from build123d import *

# Parameters (mm, degrees)
SKETCH1_W           = 133
SKETCH1_H           = 133
SKETCH1_W_2         = 125
SKETCH1_H_2         = 125
BOSS_EXTRUDE1_DEPTH = 55
SKETCH1_3_W         = 19.05
SKETCH1_3_H         = 19.05
BOSS_EXTRUDE2_DEPTH = 3.175
SKETCH2_W           = 133
SKETCH2_H           = 133
SKETCH2_R           = 2.5
BOSS_EXTRUDE3_DEPTH = 4
FILLET1_R           = 6.35
CUT_EXTRUDE1_DEPTH  = 4


with BuildPart() as part:
    # Sketch1 → Boss-Extrude1 (new body)
    with BuildSketch(Plane(origin=(0, 0, 0), x_dir=(1, 0, 0), z_dir=(0, 1, 0))):
        Rectangle(SKETCH1_W, SKETCH1_H)
        Rectangle(SKETCH1_W_2, SKETCH1_H_2, mode=Mode.SUBTRACT)
    extrude(amount=BOSS_EXTRUDE1_DEPTH)

    # Sketch1<3> → Boss-Extrude2 (add)
    with BuildSketch(Plane(origin=(0, 0, 0), x_dir=(1, 0, 0), z_dir=(0, 1, 0))):
        with Locations((-76.025, 56.975)):
            Rectangle(SKETCH1_3_W, SKETCH1_3_H)
        with Locations((-76.025, -56.975)):
            Rectangle(SKETCH1_3_W, SKETCH1_3_H)
        with Locations((76.025, -56.975)):
            Rectangle(SKETCH1_3_W, SKETCH1_3_H)
        with Locations((76.025, 56.975)):
            Rectangle(SKETCH1_3_W, SKETCH1_3_H)
    extrude(amount=BOSS_EXTRUDE2_DEPTH)

    # Sketch2 → Boss-Extrude3 (add)
    with BuildSketch(Plane(origin=(0, 55, 0), x_dir=(1, 0, 0), z_dir=(0, 1, 0))):
        Rectangle(SKETCH2_W, SKETCH2_H)
        with Locations(Location((-52.5, 52.5, 0), (0, 0, 270))):
            Circle(SKETCH2_R, mode=Mode.SUBTRACT)
        with Locations(Location((52.5, 52.5, 0), (0, 0, 270))):
            Circle(SKETCH2_R, mode=Mode.SUBTRACT)
        with Locations(Location((52.5, -52.5, 0), (0, 0, 270))):
            Circle(SKETCH2_R, mode=Mode.SUBTRACT)
        with Locations(Location((-52.5, -52.5, 0), (0, 0, 270))):
            Circle(SKETCH2_R, mode=Mode.SUBTRACT)
        Polygon((-62.5, 47.5), (-47.5, 47.5), (-47.5, 62.5), (47.5, 62.5), (47.5, 47.5), (62.5, 47.5), (62.5, -47.5), (47.5, -47.5), (47.5, -62.5), (-47.5, -62.5), (-47.5, -47.5), (-62.5, -47.5), align=None, mode=Mode.SUBTRACT)
    extrude(amount=BOSS_EXTRUDE3_DEPTH)

    # Sketch5 → CSK for 1/4 Flat Head Machine Screw (100)1 (revolve, cut)
    with BuildSketch(Plane(origin=(-76.025, 3.175, 56.975), x_dir=(0, 0, 1), z_dir=(1, 0, 0))):
        Polygon((0, 0), (0, 3.175), (3.3782, 3.175), (3.3782, 2.568232241), (6.4389, 0), align=None)
    csk_for_1_4_flat_head_machine_screw_100 = revolve(axis=Axis((-76.025, 9.525, 56.975), (0, -1, 0)), mode=Mode.SUBTRACT)

    # Mirror1: CSK for 1/4 Flat Head Machine Screw (100)1 across plane
    add(csk_for_1_4_flat_head_machine_screw_100.mirror(Plane.XY), mode=Mode.SUBTRACT)

    # Mirror1 at the second plane: CSK for 1/4 Flat Head Machine Screw (100)1 across plane
    add(csk_for_1_4_flat_head_machine_screw_100.mirror(Plane(origin=(0, 0, 0), x_dir=(0, 0, 1), z_dir=(1, 0, 0))), mode=Mode.SUBTRACT)

    # Mirror1 at the second plane copy 1 sketc → Mirror1 at the second plane copy 1 (revolve, cut)
    with BuildSketch(Plane(origin=(76.025, 3.175, -56.975), x_dir=(0, 0, -1), z_dir=(-1, 0, 0))):
        Polygon((0, 0), (0, 3.175), (3.3782, 3.175), (3.3782, 2.568232241), (6.4389, 0), align=None)
    revolve(axis=Axis((76.025, 9.525, -56.975), (0, -1, 0)), mode=Mode.SUBTRACT)

    # Fillet1
    fillet1_edges = [part.edges().sort_by_distance(p)[0] for p in [
        (-66.5, 31.0875, 66.5),
        (-66.5, 31.0875, -66.5),
        (66.5, 31.0875, -66.5),
        (66.5, 31.0875, 66.5),
        (-85.55, 1.5875, -66.5),
        (-85.55, 1.5875, -47.45),
        (-66.5, 1.5875, -47.45),
        (-85.55, 1.5875, 66.5),
        (-66.5, 1.5875, 47.45),
        (-85.55, 1.5875, 47.45),
        (85.55, 1.5875, 47.45),
        (66.5, 1.5875, 47.45),
        (85.55, 1.5875, 66.5),
        (85.55, 1.5875, -66.5),
        (66.5, 1.5875, -47.45),
        (85.55, 1.5875, -47.45),
        (-47.5, 57, -47.5),
        (-47.5, 57, 47.5),
        (47.5, 57, 47.5),
        (47.5, 57, -47.5),
    ]]
    fillet(fillet1_edges, radius=FILLET1_R)

    # Sketch6 → Cut-Extrude1 (cut)
    with BuildSketch(Plane.XY.offset(66.5)):
        with BuildLine():
            Line((44.325, 0), (44.325, 25))
            ThreePointArc((44.325, 25), (47.5, 28.175), (50.675, 25))
            Line((50.675, 25), (50.675, 0))
            ThreePointArc((50.675, 0), (47.5, -3.175), (44.325, 0))
        make_face()
    extrude(amount=-CUT_EXTRUDE1_DEPTH, mode=Mode.SUBTRACT)


solid = part.part
Input: part model. Units: mm. Frame: model coordinates. A direction names the side the tool comes from. Give positions to 0.01 mm unless a question says otherwise; leave off trailing zeros. Write each loop counter-clockwise with the first axis right and the second up, starting at its lowest first coordinate (ties: lowest second). Pieces come first, ordered by that corner, then holes. Notation, with made-up numbers: M 59,58.5 L 78,58.5 A36 cw 78,95.5 Z; hole C -16,43 d2. An arc over 180 degrees is marked long. Write item = value, one per line. Start each with the question number.
1) Cut plane D-D on z = 44. Return the cut outline in (x, y) (3 decimals), then the cut area to 3 significant figures.
2) Draft query along Z for faces 1 (the flat face through (-1, 29, 66.5)), 2 (the cylindrical face through (-64.69, 30.7, -64.59)), 3 (the flat face through (58, 57, -47.5)). Return one class per face: +Z half, -Z half, draft (parallel to the pull), parting line (faces both ways), or undercut.
3) Cut plane A-A on z = -33.5. Return the cut outline in (x, y), then the cut area to 3 significant figures.
4) Reachability of faces 4 (the cylindrical face through (68.31, 1.61, -45.54)), 5 (the flat face through (44.325, 12, 65)), 6 (the cylindrical face through (49.41, 57.03, -49.31)), 7 (the cylindrical face through (-83.64, 1.61, -49.26)) from +Z, -Z, +X, -X, +Y, -Y: full face, straight path, thin tool, end or side. Return the list, or none.
5) Material intervals for line 1 along X through (y, z) = (28, -57); line 2 along X through (y, z) = (56, 52), sorted ascending. Write a range as [from, to].
6) Cut plane C-C on y = 18. Return the cut outline in (x, z) (3 decimals), then the cut area to 3 significant figures.
7) First-contact query: pin 1 Ø2 at (y, z) = (45, 28) entering from +X; pin 2 Ø8 at (x, z) = (-76.025, -56.975) entering from +Y; pin 3 Ø4 at (x, z) = (52.5, 52.5) entering from -Y; pin 4 Ø12.5 at (x, z) = (-75, 49) entering from +Y (3 decimals). Flat tips, straight axial feed; report the tip coordinate or a pass-through.
8) Cut plane B-B on y = 32.5. Return the cut outline in (x, z), then the cut area to 3 significant figures.
Solved:
q1.outline = M -67.201,0 L -62.5,0 L -62.5,59 L -66.5,59 L -66.5,3.175 L -67.201,3.175 Z; M 62.5,0 L 67.201,0 L 67.201,3.175 L 66.5,3.175 L 66.5,59 L 62.5,59 Z
q1.area = 476 mm2
q2.face_1 = +Z half
q2.face_2 = -Z half
q2.face_3 = undercut
q3.outline = M -66.5,0 L -62.5,0 L -62.5,59 L -66.5,59 Z; M 62.5,0 L 66.5,0 L 66.5,59 L 62.5,59 Z
q3.area = 472 mm2
q4.face_4 = +X, +Y, -Y
q4.face_5 = +Z, -Y
q4.face_6 = +Y, -Y
q4.face_7 = -X, +Y, -Y
q5.line_1 = [-66.5, -62.5], [62.5, 66.5]
q5.line_2 = [-66.5, -54.95], [-50.05, -47.78], [47.78, 50.05], [54.95, 66.5]
q6.outline = M -66.5,-60.15 A6.35 ccw -60.15,-66.5 L 60.15,-66.5 A6.35 ccw 66.5,-60.15 L 66.5,60.15 A6.35 ccw 60.15,66.5 L 50.675,66.5 L 50.675,62.5 L 62.5,62.5 L 62.5,-62.5 L -62.5,-62.5 L -62.5,62.5 L 44.325,62.5 L 44.325,66.5 L -60.15,66.5 A6.35 ccw -66.5,60.15 Z
q6.area = 2,000 mm2
q7.pin_1 = 66.5
q7.pin_2 = 1.13
q7.pin_3 = through
q7.pin_4 = 3.175
q8.outline = M -66.5,-60.15 A6.35 ccw -60.15,-66.5 L 60.15,-66.5 A6.35 ccw 66.5,-60.15 L 66.5,60.15 A6.35 ccw 60.15,66.5 L -60.15,66.5 A6.35 ccw -66.5,60.15 Z; hole M -62.5,-62.5 L 62.5,-62.5 L 62.5,62.5 L -62.5,62.5 Z
q8.area = 2,030 mm2
